Input: part model. Units: mm. Frame: model coordinates. Give positions to 0.01 mm unless a question says otherwise; leave off trailing zeros. Order: outer loops, then holes, each group sorted by start corner. A loop starts at its lowest first (then second) coordinate and runs counter-clockwise, first axis right, second up.
```python
from build123d import *

# Parameters (mm, degrees)
BOSS_EXTRUDE2_DEPTH = 400
CUT_EXTRUDE1_DEPTH  = 100


with BuildPart() as part:
    # Sketch1 → Boss-Extrude2 (new body)
    with BuildSketch(Plane.XY):
        with BuildLine():
            Line((0, 0), (-11.7, 0))
            ThreePointArc((-11.7, 0), (-12.972792206, 0.527207794), (-13.5, 1.8))
            Line((-13.5, 1.8), (-13.5, 6.7))
            ThreePointArc((-13.5, 6.7), (-13.734314575, 7.265685425), (-14.3, 7.5))
            Line((-14.3, 7.5), (-17.5, 7.5))
            Line((-17.5, 7.5), (-17.5, 8.5))
            Line((-17.5, 8.5), (-14.3, 8.5))
            ThreePointArc((-14.3, 8.5), (-13.027207794, 7.972792206), (-12.5, 6.7))
            Line((-12.5, 6.7), (-12.5, 1.8))
            ThreePointArc((-12.5, 1.8), (-12.265685425, 1.234314575), (-11.7, 1))
            Line((-11.7, 1), (0, 1))
            Line((0, 1), (11.7, 1))
            ThreePointArc((11.7, 1), (12.265685425, 1.234314575), (12.5, 1.8))
            Line((12.5, 1.8), (12.5, 6.7))
            ThreePointArc((12.5, 6.7), (13.027207794, 7.972792206), (14.3, 8.5))
            Line((14.3, 8.5), (17.5, 8.5))
            Line((17.5, 8.5), (17.5, 7.5))
            Line((17.5, 7.5), (14.3, 7.5))
            ThreePointArc((14.3, 7.5), (13.734314575, 7.265685425), (13.5, 6.7))
            Line((13.5, 6.7), (13.5, 1.8))
            ThreePointArc((13.5, 1.8), (12.972792206, 0.527207794), (11.7, 0))
            Line((11.7, 0), (0, 0))
        make_face()
    extrude(amount=BOSS_EXTRUDE2_DEPTH)

    # Sketch2 → Cut-Extrude1 (cut)
    with BuildSketch(Plane(origin=(0, 1, 0), x_dir=(1, 0, 0), z_dir=(0, 1, 0))):
        with BuildLine():
            Line((-3.1, -390), (-3.1, -375))
            ThreePointArc((-3.1, -375), (0, -371.9), (3.1, -375))
            Line((3.1, -375), (3.1, -390))
            ThreePointArc((3.1, -390), (0, -393.1), (-3.1, -390))
        make_face()
        with BuildLine():
            Line((-3.1, -365), (-3.1, -350))
            ThreePointArc((-3.1, -350), (0, -346.9), (3.1, -350))
            Line((3.1, -350), (3.1, -365))
            ThreePointArc((3.1, -365), (0, -368.1), (-3.1, -365))
        make_face()
        with BuildLine():
            Line((-3.1, -340), (-3.1, -325))
            ThreePointArc((-3.1, -325), (0, -321.9), (3.1, -325))
            Line((3.1, -325), (3.1, -340))
            ThreePointArc((3.1, -340), (0, -343.1), (-3.1, -340))
        make_face()
        with BuildLine():
            Line((-3.1, -315), (-3.1, -300))
            ThreePointArc((-3.1, -300), (0, -296.9), (3.1, -300))
            Line((3.1, -300), (3.1, -315))
            ThreePointArc((3.1, -315), (0, -318.1), (-3.1, -315))
        make_face()
        with BuildLine():
            Line((-3.1, -415), (-3.1, -400))
            ThreePointArc((-3.1, -400), (0, -396.9), (3.1, -400))
            Line((3.1, -400), (3.1, -415))
            ThreePointArc((3.1, -415), (0, -418.1), (-3.1, -415))
        make_face()
        with BuildLine():
            Line((-3.1, -290), (-3.1, -275))
            ThreePointArc((-3.1, -275), (0, -271.9), (3.1, -275))
            Line((3.1, -275), (3.1, -290))
            ThreePointArc((3.1, -290), (0, -293.1), (-3.1, -290))
        make_face()
        with BuildLine():
            Line((-3.1, -265), (-3.1, -250))
            ThreePointArc((-3.1, -250), (0, -246.9), (3.1, -250))
            Line((3.1, -250), (3.1, -265))
            ThreePointArc((3.1, -265), (0, -268.1), (-3.1, -265))
        make_face()
        with BuildLine():
            Line((-3.1, -240), (-3.1, -225))
            ThreePointArc((-3.1, -225), (0, -221.9), (3.1, -225))
            Line((3.1, -225), (3.1, -240))
            ThreePointArc((3.1, -240), (0, -243.1), (-3.1, -240))
        make_face()
        with BuildLine():
            Line((-3.1, -215), (-3.1, -200))
            ThreePointArc((-3.1, -200), (0, -196.9), (3.1, -200))
            Line((3.1, -200), (3.1, -215))
            ThreePointArc((3.1, -215), (0, -218.1), (-3.1, -215))
        make_face()
        with BuildLine():
            Line((-3.1, -190), (-3.1, -175))
            ThreePointArc((-3.1, -175), (0, -171.9), (3.1, -175))
            Line((3.1, -175), (3.1, -190))
            ThreePointArc((3.1, -190), (0, -193.1), (-3.1, -190))
        make_face()
        with BuildLine():
            Line((-3.1, -165), (-3.1, -150))
            ThreePointArc((-3.1, -150), (0, -146.9), (3.1, -150))
            Line((3.1, -150), (3.1, -165))
            ThreePointArc((3.1, -165), (0, -168.1), (-3.1, -165))
        make_face()
        with BuildLine():
            Line((-3.1, -140), (-3.1, -125))
            ThreePointArc((-3.1, -125), (0, -121.9), (3.1, -125))
            Line((3.1, -125), (3.1, -140))
            ThreePointArc((3.1, -140), (0, -143.1), (-3.1, -140))
        make_face()
        with BuildLine():
            Line((-3.1, -115), (-3.1, -100))
            ThreePointArc((-3.1, -100), (0, -96.9), (3.1, -100))
            Line((3.1, -100), (3.1, -115))
            ThreePointArc((3.1, -115), (0, -118.1), (-3.1, -115))
        make_face()
        with BuildLine():
            Line((-3.1, -90), (-3.1, -75))
            ThreePointArc((-3.1, -75), (0, -71.9), (3.1, -75))
            Line((3.1, -75), (3.1, -90))
            ThreePointArc((3.1, -90), (0, -93.1), (-3.1, -90))
        make_face()
        with BuildLine():
            Line((-3.1, -65), (-3.1, -50))
            ThreePointArc((-3.1, -50), (0, -46.9), (3.1, -50))
            Line((3.1, -50), (3.1, -65))
            ThreePointArc((3.1, -65), (0, -68.1), (-3.1, -65))
        make_face()
        with BuildLine():
            Line((-3.1, -40), (-3.1, -25))
            ThreePointArc((-3.1, -25), (0, -21.9), (3.1, -25))
            Line((3.1, -25), (3.1, -40))
            ThreePointArc((3.1, -40), (0, -43.1), (-3.1, -40))
        make_face()
        with BuildLine():
            Line((-3.1, -15), (-3.1, 0))
            ThreePointArc((-3.1, 0), (0, 3.1), (3.1, 0))
            Line((3.1, 0), (3.1, -15))
            ThreePointArc((3.1, -15), (0, -18.1), (-3.1, -15))
        make_face()
    extrude(amount=-CUT_EXTRUDE1_DEPTH, mode=Mode.SUBTRACT)


solid = part.part
```
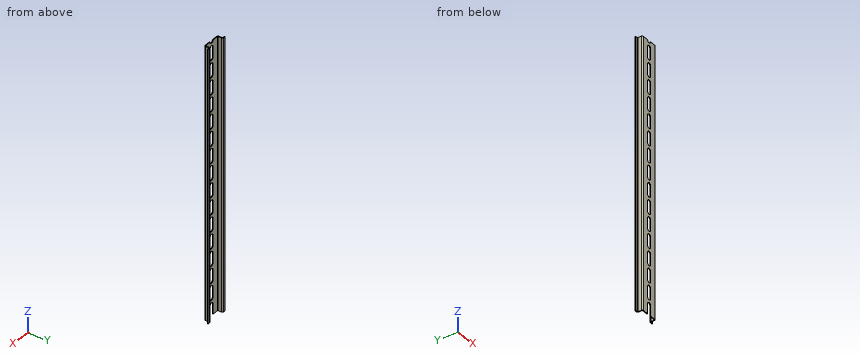
1) Line query: probe 1 along X at (y, z) = (3, 142.5); probe 2 along X at (y, z) = (1.5, 352); probe 3 along Y at (x, z) = (-6, 204.5). Output: solid intervals per line, ascending.
2) Cut plane A-A (z = 328.5). Return the cut outline in (x, y), then the cut area to 3 significant figures.
3) First-contact query: P1, Ø1, axis at x = 13, z = 252.5, coming from the -Y side; P2, Ø0.8, axis at y = 0.5, z = 279.5, coming from the -X side; P3, Ø1.5, axis at y = 4.5, z = 239.5, coming from the +X side. Flat tips, straight axial feed; report the tip coordinate or a pass-through.
Geometry says:
1. probe 1: x = -13.5 to -12.5, 12.5 to 13.5
1. probe 2: x = -13.47 to -12.44, 12.44 to 13.47
1. probe 3: y = 0 to 1
2. outline: (-17.5, 7.5) - (-14.3, 7.5) arc R0.8 cw to (-13.5, 6.7) - (-13.5, 1.8) arc R1.8 ccw to (-11.7, 0) - (-3.1, 0) - (-3.1, 1) - (-11.7, 1) arc R0.8 cw to (-12.5, 1.8) - (-12.5, 6.7) arc R1.8 ccw to (-14.3, 8.5) - (-17.5, 8.5) - close; (3.1, 0) - (11.7, 0) arc R1.8 ccw to (13.5, 1.8) - (13.5, 6.7) arc R0.8 cw to (14.3, 7.5) - (17.5, 7.5) - (17.5, 8.5) - (14.3, 8.5) arc R1.8 ccw to (12.5, 6.7) - (12.5, 1.8) arc R0.8 cw to (11.7, 1) - (3.1, 1) - close
2. area: 41.6 mm2
3. P1: stops at y = 0.19
3. P2: stops at x = -13.26
3. P3: stops at x = 13.5
